Geometry check sheet. Reference: the model listing, model coordinates, mm. A direction names the side the tool comes from. Give positions to 0.01 mm unless a question says otherwise; leave off trailing zeros. Loops run counter-clockwise (first coordinate to the right, second up) from the corner with the lowest first, then second, coordinate; pieces in that order, holes last. Notation, with made-up numbers: (31, -32) -> (43, -32) arc R16 ccw to (43, -22) -> close; hole circle Ø1 at (83.5, -7). An arc over 180 degrees is marked (long way). One line per question, with ' | ' between items.
Autodesk Inventor part; units mm, degrees
ref_plane "YZ Plane" through (0, 0, 0) normal (1, 0, 0) x (0, 1, 0)
ref_plane "XZ Plane" through (0, 0, 0) normal (0, 1, 0) x (-1, 0, 0)
ref_plane "XY Plane" through (0, 0, 0) normal (0, 0, 1) x (1, 0, 0)
sketch "Sketch1" plane through (0, 0, 0) normal (0, 0, 1) x (1, 0, 0)
  line L0 (-10, -10) -> (10, -10)
  line L1 (10, -10) -> (10, 10)
  line L2 (10, 10) -> (-10, 10)
  line L3 (-10, 10) -> (-10, -10)
  line L4 (-10, -10) -> (10, 10) construction
  line L5 (10, -10) -> (-10, 10) construction
  line L6 (7, 10) -> (7, -10)
  circle A0 centre (3, 0) radius 3
  circle A1 centre (-5, 0) radius 3
  line L7 (-5, 3) -> (3, 3)
  line L8 (-5, -3) -> (3, -3)
  line L9 (10, -10) -> (10, 17.1252) construction
  line L10 (7, 8) -> (-10, 8)
  line L11 (7, -8) -> (-10, -8)
  point P0 (0, 0)
  dimension "d0" = 20
  dimension "d1" = 20
  dimension "d2" = 3
  dimension "d3" = 6
  dimension "d4" = 4
  dimension "d5" = 6
  dimension "d6" = 5
  dimension "d16" = 2
  dimension "d17" = 2
extrude "Extrusion1" add sketch "Sketch1" against normal blind 3 contours L3 L11 L6 L0 | L6 L2 L1 L0 | L3 L10 L6 L11 | L3 L2 L6 L10 | A0 | A0 L8 A1 L7 | A1
extrude "Extrusion2" add sketch "Sketch1" along normal blind 17 contours L6 L2 L1 L0
sketch "Sketch2" plane through (-10, -10, -3) normal (0, -1, 0) x (1, 0, 0)
  line L0 (0, 3) -> (17, 3)
  line L1 (17, 3) -> (7, 3)
  line L2 (17, 3) -> (17, 20)
  line L3 (17, 13) -> (17, 3)
  line L4 (17, 13) -> (7, 3)
  point P0 (10, 3)
  dimension "d11" = 10
  dimension "d13" = 10
extrude "Extrusion3" add sketch "Sketch2" against normal blind 20
extrude "Extrusion4" cut sketch "Sketch1" along normal blind 20 contours L3 L10 L6 L11 | A0 | A0 L8 A1 L7 | A1
sketch "Sketch3" plane through (7, -10, 17) normal (-1, 0, 0) x (0, 0, 1)
  circle A0 centre (-4.9998, 10.0301) radius 3
  circle A1 centre (-12.9998, 10.0301) radius 3
  line L0 (-12.9998, 13.0301) -> (-4.9998, 13.0301)
  line L1 (-12.9998, 7.0301) -> (-4.9998, 7.0301)
  line L2 (0, 20) -> (0, 0)
  line L3 (0, 10) -> (-2, 10) construction
  point P0 (-17, 10)
  dimension "d20" = 6
  dimension "d21" = 6
  dimension "d22" = 2
extrude "Extrusion5" cut sketch "Sketch1" against normal blind 3 contours A0 | A0 L8 A1 L7 | A1
extrude "Extrusion6" cut sketch "Sketch3" against normal blind 3
fillet "Fillet1" radius 1 8 edges at (8.5, -10, 17) (8.5, 10, 17) (7, 0, 17) (10, 0, 17) (-10, 0, 0) (-10, 0, -3) (-10, 10, -1.5) (-10, -10, -1.5)
properties part number "grid_board_8020_corner_mount"
Item 1: Scan lines: probe 1 along Y at (x, z) = (-1.5, -1); probe 2 along X at (y, z) = (4.25, 12.5); probe 3 along Z at (x, y) = (-7.75, -5). Record each from-to range of solid material in increasing order.
Result:
probe 1: -10 to -3, 3 to 10 | probe 2: 7 to 10 | probe 3: -3 to 0
Item 2: Sectioned sample at C-C (y = -1.5). Record the cut outline in (x, z), plus the area to 3 significant figures.
Result:
outline: (-10, -2) arc R1 ccw to (-9, -3) -> (-7.6, -3) -> (-7.6, 0) -> (-9, 0) arc R1 ccw to (-10, -1) -> close; (5.6, -3) -> (10, -3) -> (10, 1.42) -> (7, 1.42) -> (7, 0) -> (5.6, 0) -> close; (7, 14.58) -> (10, 14.58) -> (10, 16) arc R1 ccw to (9, 17) -> (8, 17) arc R1 ccw to (7, 16) -> close | area: 31.1 mm2
Item 3: Sectioned sample at D-D (x = 6.5). Record the cut outline in (y, z), plus the area to 3 significant figures.
Result:
outline: (-10, -3) -> (10, -3) -> (10, 9.5) -> (8, 9.5) -> (8, 0) -> (-8, 0) -> (-8, 9.5) -> (-10, 9.5) -> close | area: 98.0 mm2
Item 4: Release check for a two-part mould opening along Y. For faces 1 (the face through (5, -10, 2)), 2 (the face through (8, 0, 1)), 3 (the face through (0, 5, -3)) record: pulls with the +Y half, pulls with the -Y half, needs draft (parallel to the pull), parting line crosses it, or undercut.
Result:
face 1: pulls with the -Y half | face 2: undercut | face 3: needs draft
Item 5: Set-up check for faces 4 (the face through (9.699, 0.14, 16.715)), 5 (the face through (7, -4, 8)), 6 (the face through (-9.699, -0.14, -0.285)), 7 (the face through (8, 3.03, 8)), 8 (the face through (-8, 0, -1)): record each of +Z, -Z, +X, -X, +Y, -Y from which the full face is reachable in a straight line by a thin tool's end or side.
Result:
face 4: +Z, +X, +Y, -Y | face 5: +Z, -X | face 6: +Z, -X, +Y, -Y | face 7: +X, -X | face 8: +Z, -Z
Item 6: Depth check by flat-ended pin: pin 1 Ø5 at (x, y) = (1, -3) entering from +Z; pin 2 Ø5 at (y, z) = (-3, 14) entering from -X. Enter the tip coordinate at first touch or a pass-through.
Result:
pin 1: z = 0 | pin 2: x = 7
Item 7: Sectioned sample at A-A (z = 7.25). Record the cut outline in (x, y).
Result:
outline: (4.25, -10) -> (10, -10) -> (10, -2.97) -> (7, -2.97) -> (7, -8) -> (4.25, -8) -> close; (4.25, 8) -> (7, 8) -> (7, 3.03) -> (10, 3.03) -> (10, 10) -> (4.25, 10) -> close
Item 8: Sectioned sample at B-B (x = -2.5). Record the cut outline in (y, z).
Result:
outline: (-10, -3) -> (-3, -3) -> (-3, 0) -> (-8, 0) -> (-8, 0.5) -> (-10, 0.5) -> close; (3, -3) -> (10, -3) -> (10, 0.5) -> (8, 0.5) -> (8, 0) -> (3, 0) -> close
